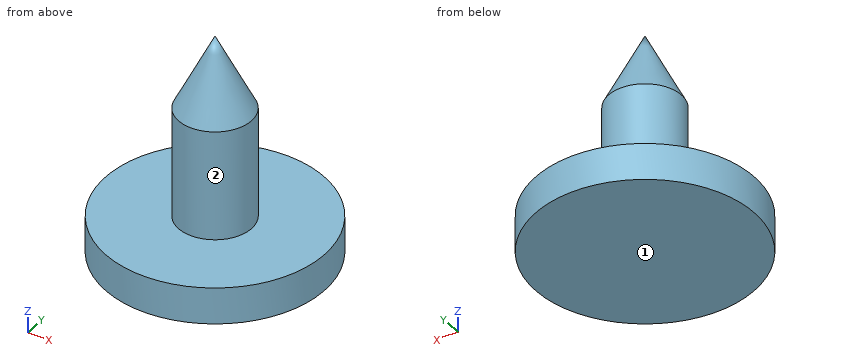
from build123d import *

# Parameters (mm, degrees)
CYLINDER_R        = 3
CYLINDER_DEPTH    = 1
CYLINDER001_R     = 1
CYLINDER001_DEPTH = 4


with BuildPart() as part:
    # Cylinder → Cylinder (join)
    with BuildSketch(Plane.XY):
        Circle(CYLINDER_R)
    extrude(amount=CYLINDER_DEPTH)

    # Cylinder001 → Cylinder001 (join)
    with BuildSketch(Plane.XY):
        Circle(CYLINDER001_R)
    extrude(amount=CYLINDER001_DEPTH)

    # Cone → Cone (revolve)
    with BuildSketch(Plane(origin=(0, 0, 4), x_dir=(1, 0, 0), z_dir=(0, -1, 0))):
        Polygon((0, 0), (1, 0), (0, 2), align=None)
    revolve(axis=Axis((0, 0, 4), (0, 0, 1)))


solid = part.part
The listing builds one solid part. Answer for the finished solid, in the listing's coordinates (mm). Face numbers are marked on the shaded views. A direction names the side the tool comes from. Give positions to 0.01 mm unless a question says otherwise; leave off trailing zeros. Write each loop counter-clockwise with the first axis right and the second up, starting at its lowest first coordinate (ties: lowest second). Pieces come first, ordered by that corner, then holes. Notation, with made-up numbers: (3, 75) - (15, 75) arc R26 cw to (15, 99) - close; hole circle Ø9 at (25.25, -13.5). An arc over 180 degrees is marked (long way). One line per question, with ' | ' between items. Start each with the question number.
1. Section A-A, the plane z = 3.8 is taken. Determine the outline of the cut face in (x, y), then the cut area to 3 significant figures.
2. Given P1, Ø1.5, axis at y = 2.5, z = 3.5, coming from the +X side; P2, Ø3, axis at x = 0.5, y = -1, coming from the -Z side; P3, Ø1, axis at y = 0, z = 5, coming from the -X side, each flat-ended and moving along its own axis, determine where each tip first touches the part or whether it passes through.
3. Section C-C, the plane x = 1.9 is taken. Determine the outline of the cut face in (y, z), then the cut area to 3 significant figures.
4. Section B-B, the plane y = 1.1 is taken. Determine the outline of the cut face in (x, z), then the cut area to 3 significant figures.
5. For the marked faces 1 and 2, determine the directions among +Z, -Z, +X, -X, +Y, -Y from which every point of the face is accessible in a straight line to the end or side of a thin tool.
6. Straight lines are drawn through the part: line 1 (Z direction, x = 0.8, y = -0.9); line 2 (Y direction, x = 0.15, z = 4.25); line 3 (Y direction, x = 0.6, z = 4.25). For each, find the intervals that lie inside material, in ascending order.
7. Section D-D, the plane z = 5.05 is taken. Determine the outline of the cut face in (x, y) (3 decimals).
Result:
1) outline: circle Ø2 at (0, 0) | area: 3.14 mm2
2) P1: passes through | P2: stops at z = 0 | P3: stops at x = -0.75
3) outline: (-2.32, 0) - (2.32, 0) - (2.32, 1) - (-2.32, 1) - close | area: 4.64 mm2
4) outline: (-2.79, 0) - (2.79, 0) - (2.79, 1) - (-2.79, 1) - close | area: 5.58 mm2
5) face 1: -Z, +X, -X, +Y, -Y | face 2: +Z
6) line 1: z = 0 to 1 | line 2: y = -0.86 to 0.86 | line 3: y = -0.64 to 0.64
7) outline: circle Ø0.95 at (0, 0)
